Verification items for the finished model (mm, model axes). A direction names the side the tool comes from. Round coordinates to 2 decimals unless told otherwise and drop trailing zeros. Loops run counter-clockwise (first coordinate to the right, second up) from the corner with the lowest first, then second, coordinate; pieces in that order, holes last. Notation, with made-up numbers: (4.25, 38.5) -> (51.25, 38.5) arc R8 cw to (51.25, 49.5) -> close; hole circle Ø10 at (1.5, 18). An arc over 180 degrees is marked (long way). Use CSV: the item, a comma, the result in double quotes. Start each with the question number.
```python
from build123d import *

# Parameters (mm, degrees)
CUT_EXTRUDE_2_DEPTH      = 17
CHAMFER_1_SIZE           = 1
SKETCH_5_OUTSIDE_W       = 32.926
SKETCH_5_OUTSIDE_H       = 32.926
CUT_EXTRUDE_4_DEPTH      = 1.7
CUT_EXTRUDE_5_DEPTH      = 36.580893749
CUT_EXTRUDE_5_DEPTH_BACK = 36.580893749


# Read off the part's stored shape, not the designer's step: Диаметр отверстия Ø2.3 (2.3)1
with BuildPart() as part:
    # Эскиз1 → Повернуть1 (revolve)
    with BuildSketch(Plane.XY, mode=Mode.PRIVATE) as revolve_1_sk:
        Polygon((5.85, 0), (5.85, 11), (6, 11), (6, 32), (11, 32), (11, 13), (7.5, 13), (7.5, 0), align=None)
    revolve(revolve_1_sk.sketch.rotate(Axis((0, 0, 0), (0, 1, 0)), 90), axis=Axis((0, 0, 0), (0, 1, 0)))

    # Эскиз2 → Вырез-Вытянуть2 (cut)
    with BuildSketch(Plane(origin=(0, 32, 0), x_dir=(1, 0, 0), z_dir=(0, 1, 0))):
        with BuildLine():
            Line((-5.196152423, 3), (-10.583005244, 3))
            ThreePointArc((-10.583005244, 3), (-1.514421063, -10.895252583), (11, 0))
            ThreePointArc((11, 0), (3.74273909, 10.343689096), (-8.453073474, 7.038859911))
            Line((-8.453073474, 7.038859911), (-4.890406914, 3.476193351))
            ThreePointArc((-4.890406914, 3.476193351), (1.824494247, 5.715874451), (6, 0))
            ThreePointArc((6, 0), (-1.552914271, -5.795554958), (-5.196152423, 3))
        make_face()
    extrude(amount=-CUT_EXTRUDE_2_DEPTH, mode=Mode.SUBTRACT)

    # Фаска1
    chamfer_1_edges = [part.edges().sort_by_distance(p)[0] for p in [
        (0, 13, 11),
    ]]
    chamfer(chamfer_1_edges, length=CHAMFER_1_SIZE)

    # Эскиз5 outside → Вырез-Вытянуть4 (cut)
    with BuildSketch(Plane.XZ):
        Rectangle(SKETCH_5_OUTSIDE_W, SKETCH_5_OUTSIDE_H)
        with BuildLine():
            Line((0, 0), (3.954322794, 1))
            Line((3.954322794, 1), (7.433034374, 1))
            ThreePointArc((7.433034374, 1), (7.5, 0), (7.433034374, -1))
            Line((7.433034374, -1), (3.955330555, -1))
            Line((3.955330555, -1), (0, 0))
        make_face(mode=Mode.SUBTRACT)
    extrude(amount=-CUT_EXTRUDE_4_DEPTH, mode=Mode.SUBTRACT)

    # Эскиз6 → Вырез-Вытянуть5 (cut, two sides: drawn at the far end of the back side and taken through both)
    with BuildSketch(Plane(origin=(0, 0, 0), x_dir=(0, 0, -1), z_dir=(1, 0, 0)).offset(-CUT_EXTRUDE_5_DEPTH_BACK)):
        Polygon((82.137450445, 10.5), (7.5, 10.5), (7, 10.5), (7, 5.5), (7.5, 5.5), (82.137450445, 5.5), (231.412351334, 5.5), (231.412351334, 10.5), align=None)
    extrude(amount=CUT_EXTRUDE_5_DEPTH + CUT_EXTRUDE_5_DEPTH_BACK, mode=Mode.SUBTRACT)

    # Диаметр отверстия Ø2.3 (2.3)1 outline → Диаметр отверстия Ø2.3 (2.3)1 (revolve, cut)
    with BuildSketch(Plane.XZ.offset(-8)):
        Polygon((1.15, -6.9), (1.15, -5.735802951), (0, -5.735802951), (0, -7), (1.25, -7), align=None)
    revolve(axis=Axis((0, 8, 0), (0, 0, 1)), mode=Mode.SUBTRACT)


solid = part.part
```
Q1. Cross-section at A-A (x = 0). Record the boundary of the cut face in (y, z).
Q2. Cross-section at C-C (z = 0). Record the boundary of the cut face in (x, y).
Q3. Depth check by flat-ended pin: pin 1 Ø3 at (x, y) = (-2, 21) entering from -Z; pin 2 Ø5 at (x, y) = (4, 8.5) entering from -Z; pin 3 Ø2.5 at (x, y) = (-8, 24) entering from +Z; pin 4 Ø0.6 at (x, z) = (0.5, -7.5) entering from +Y. Enter the tip coordinate at first touch or a pass-through.
Q4. Cross-section at D-D (y = 3.5). Record the boundary of the cut face in (x, z), and give its area (3 significant figures).
Q5. Tool access check on faces 5 (the face through (-1.15, 8.05, -6.31)), 6 (the face through (-7, 13, -4)), 7 (the face through (-8, 24, -3)), 8 (the face through (7, 1, -1)). Record the directions out of +Z, -Z, +X, -X, +Y, -Y that give a thin tool (end or side, any length) a straight path to the whole face; none if there is none.
Q6. Thickness scan on L1, parallel to X at y = 4.75, z = 0; L2, parallel to Y at x = 0.75, z = 9.75; L3, parallel to X at y = 8, z = -6.6. Record the ranges inside material, lowest first. Write a range as from..to.
Q7. Cross-section at B-B (y = 8). Record the boundary of the cut face in (x, z).
Q8. Release check for a two-part mould opening along Z. For faces 1 (the face through (7, 1, 1)), 2 (the face through (5.19, 6.8, -2.7)), 3 (the face through (-6, 1.7, -2)), 4 (the face through (-1, 9, -7)) record: +Z half, -Z half, draft (parallel to the pull), parting line (faces both ways), or undercut.
Answer list:
1,outline,"(1.7, -7.5) -> (5.5, -7.5) -> (5.5, -7) -> (6.75, -7) -> (6.85, -6.9) -> (6.85, -5.85) -> (1.7, -5.85) -> close; (1.7, 5.85) -> (11, 5.85) -> (11, 6) -> (15, 6) -> (15, 11) -> (14, 11) -> (13, 10) -> (13, 7.5) -> (1.7, 7.5) -> close; (9.15, -6.9) -> (9.25, -7) -> (10.5, -7) -> (10.5, -7.5) -> (13, -7.5) -> (13, -10) -> (14, -11) -> (15, -11) -> (15, -6) -> (11, -6) -> (11, -5.85) -> (9.15, -5.85) -> close"
2,outline,"(-11, 14) -> (-10, 13) -> (-7.5, 13) -> (-7.5, 1.7) -> (-5.85, 1.7) -> (-5.85, 11) -> (-6, 11) -> (-6, 15) -> (-11, 15) -> close; (5.85, 0) -> (7.5, 0) -> (7.5, 13) -> (10, 13) -> (11, 14) -> (11, 15) -> (6, 15) -> (6, 11) -> (5.85, 11) -> close"
3,pin 1,"passes through"
3,pin 2,"stops at z = -7.07"
3,pin 3,"stops at z = -3"
3,pin 4,"stops at y = 15"
4,outline,"circle Ø15 at (0, 0); hole circle Ø11.7 at (0, 0)"
4,area,"69.2 mm2"
5,face 5,"-Z"
5,face 6,"-Y"
5,face 7,"+Z, +X, -X, +Y"
5,face 8,"-Z, +X, -X, -Y"
6,L1,"x = -7.5..-5.85, 5.85..7.5"
6,L2,"y = 13..15"
6,L3,"x = -3.56..-1.15, 1.15..3.56"
7,outline,"(-2.69, -7) -> (-1.25, -7) -> (-1.15, -6.9) -> (-1.15, -5.74) arc R5.85 cw (long way) to (1.15, -5.74) -> (1.15, -6.9) -> (1.25, -7) -> (2.69, -7) arc R7.5 ccw (long way) to start"
8,face 1,"+Z half"
8,face 2,"undercut"
8,face 3,"draft"
8,face 4,"-Z half"
